For this review, take the finished solid that the model builds, in its own axes (mm). A direction names the side the tool comes from. Coordinates: 2 decimals unless noted, no trailing zeros. Loops run counter-clockwise (first coordinate to the right, second up) from the corner with the lowest first, then second, coordinate; pieces in that order, holes last. Notation, with made-up numbers: (2, 40) -> (28, 40) arc R31 cw to (28, 71) -> close; hole circle Ø4 at (65, 3). An arc over 180 degrees is marked (long way). One line per item, written item: value.
from build123d import *

# Parameters (mm, degrees)
SKETCH_1_R          = 2.75
SKETCH_1_R_2        = 1.5
EXTRUDE_397_DEPTH   = 2
SKETCH_1_3_R        = 1.5
EXTRUDE_432_DEPTH   = 12
CUT_EXTRUDE_1_DEPTH = 1.3


with BuildPart() as part:
    # Sketch 1 → Extrude 397 (new body)
    # profile 1 of 2: a face of its own
    with BuildSketch(Plane(origin=(0, 0, 0), x_dir=(1, 0, 0), z_dir=(0, 1, 0))):
        with Locations(Location((0, 0, 0), (0, 0, 270))):
            Circle(SKETCH_1_R)
        Circle(SKETCH_1_R_2, mode=Mode.SUBTRACT)
    # profile 2 of 2: a face of its own
    with BuildSketch(Plane(origin=(0, 0, 0), x_dir=(1, 0, 0), z_dir=(0, 1, 0))):
        Circle(SKETCH_1_R_2)
    extrude(amount=EXTRUDE_397_DEPTH)

    # Sketch 1_3 → Extrude 432 (add)
    with BuildSketch(Plane(origin=(0, 0, 0), x_dir=(1, 0, 0), z_dir=(0, 1, 0))):
        with Locations(Location((0, 0, 0), (0, 0, 270))):
            Circle(SKETCH_1_3_R)
    extrude(amount=-EXTRUDE_432_DEPTH)

    # Sketch 2 → Cut-Extrude 1 (cut)
    with BuildSketch(Plane(origin=(0, 2, 0), x_dir=(1, 0, 0), z_dir=(0, 1, 0))):
        Polygon((1.443375673, 0), (0.721687836, 1.25), (-0.721687836, 1.25), (-1.443375673, 0), (-0.721687836, -1.25), (0.721687836, -1.25), align=None)
    extrude(amount=-CUT_EXTRUDE_1_DEPTH, mode=Mode.SUBTRACT)


solid = part.part
1. The part is to be moulded in two halves that separate along X. For faces 1 (the flat face through (0, 0.7, 0)), 2 (the flat face through (1.3, 2, 0.6)), 3 (the cylindrical face through (0.45, -5.92, 1.43)), say which applies: pulls with the +X half, pulls with the -X half, needs draft (parallel to the pull), parting line crosses it, or undercut.
Return value:
face 1: undercut
face 2: needs draft
face 3: parting line crosses it
2. Take a section at C-C, the plane y = -2.5. Give the boundary of the cut face in (x, z), and give its area (3 significant figures).
Return value:
outline: circle Ø3 at (0, 0)
area: 7.07 mm2
3. Take a section at B-B, the plane x = 0. Give the boundary of the cut face in (y, z).
Return value:
outline: (-12, -1.5) -> (0, -1.5) -> (0, -2.75) -> (2, -2.75) -> (2, -1.25) -> (0.7, -1.25) -> (0.7, 1.25) -> (2, 1.25) -> (2, 2.75) -> (0, 2.75) -> (0, 1.5) -> (-12, 1.5) -> close
4. Take a section at A-A, the plane y = 1.25. Give the boundary of the cut face in (x, z).
Return value:
outline: circle Ø5.5 at (0, 0); hole (-1.44, 0) -> (-0.72, -1.25) -> (0.72, -1.25) -> (1.44, 0) -> (0.72, 1.25) -> (-0.72, 1.25) -> close
5. For faces 4 (the flat face through (0, -12, 0)), 5 (the flat face through (1.2, 0, 1.2)), 6 (the flat face through (1.08, 1.36, 0.63)), list the 3-axis set-ups (+Z, -Z, +X, -X, +Y, -Y) from which the entire face can be reached by the end or side of a thin tool; tool diameter is ignored.
Return value:
face 4: +Z, -Z, +X, -X, -Y
face 5: -Y
face 6: +Y
6. Take a section at D-D, the plane z = 1.05. Give the boundary of the cut face in (x, y), and give its area (3 significant figures).
Return value:
outline: (-2.54, 0) -> (-1.07, 0) -> (-1.07, -12) -> (1.07, -12) -> (1.07, 0) -> (2.54, 0) -> (2.54, 2) -> (0.84, 2) -> (0.84, 0.7) -> (-0.84, 0.7) -> (-0.84, 2) -> (-2.54, 2) -> close
area: 33.7 mm2
7. Insertion check: pin 1 Ø1.5 at (y, z) = (-5, -1.5) entering from +X; pin 2 Ø1 at (y, z) = (-10, 0.5) entering from +X. Each pin has a flat end and moves straight along its axis. Give the tip position at first contact, or say it passes through.
Return value:
pin 1: stops at x = 1.3
pin 2: stops at x = 1.5
8. To check wall thickness, follow probe 1 along Y at (x, z) = (-2.4, 1.2); probe 2 along Y at (x, z) = (0.95, -0.3); probe 3 along X at (y, z) = (-8, -0.05). State the ranges of each line that lie inside material, in increasing order. Write a range as from..to.
Return value:
probe 1: y = 0..2
probe 2: y = -12..0.7
probe 3: x = -1.5..1.5
